Check sheet for the modelled part. Datum: model origin and axes. Units: mm. A direction names the side the tool comes from. Give positions to 0.01 mm unless a question says otherwise; leave off trailing zeros. Write each loop counter-clockwise with the first axis right and the second up, starting at its lowest first coordinate (ties: lowest second). Pieces come first, ordered by that corner, then holes. Notation, with made-up numbers: (-10, -36.75) -> (0, -36.75) arc R16 ccw to (0, -17.75) -> close; hole circle Ø7 at (84.25, 6). An arc over 180 degrees is marked (long way). Use a Markdown table: item, result. Add a question column.
1. Cross-section at A-A (x = 2). Enter the section's corners in (y, z).
2. Release check for a two-part mould opening along Y. For faces 4 (the cylindrical face through (4.5, 23.6, 3.6)), 5 (the flat face through (0.1, 0, 4.3)), 6 (the cylindrical face through (4.5, 23.6, -3.7)), 7 (the cylindrical face through (-0.1, 26.1, 2.5)) record: released by +Y, released by -Y, zero draft, split by the parting line, or undercut.
3. Set-up check for faces 1 (the flat face through (0, 17.5, 3)), 2 (the cylindrical face through (0.1, 26.1, -2.5)), 3 (the flat face through (6, 18, -0.25)): record each of +Z, -Z, +X, -X, +Y, -Y from which the full face is reachable in a straight line by a thin tool's end or side.
4. Cross-section at D-D (y = 14). Enter the section's corners in (x, z), then the cut area to 3 significant figures.
5. Cross-section at C-C (z = 8). Enter the section's corners in (x, y).
6. Cross-section at B-B (y = 31.5). Enter the section's corners in (x, z).
7. Scan lines: probe 1 along X at (y, z) = (3.5, 3.25); probe 2 along Y at (x, z) = (7.5, -2.75); probe 3 along Z at (x, y) = (4.5, 10.5). Record each from-to range of solid material in increasing order. Write a range as [from, to].
8. Gauge pin test, flat ends, axial feed: P1, Ø3.5, axis at x = 6.5, y = 3.5, coming from the +Z side; P2, Ø10, axis at x = 7.5, y = 29, coming from the +Z side; P3, Ø1.9, axis at x = 1.5, z = 3, coming from the -Y side; P4, Ø1.3, axis at x = -3.5, y = 15.5, coming from the +Z side. Record the tip position at first contact, or that the pin passes through.
from build123d import *

# Parameters (mm, degrees)
SKETCH1_R               = 10
BOSS_EXTRUDE1_DEPTH     = 35
CUT_EXTRUDE1_DEPTH      = 38.749172176
CUT_EXTRUDE1_DEPTH_BACK = 38.749172176
SKETCH2_R               = 2.5
SKETCH3_R               = 4
CUT_EXTRUDE2_DEPTH      = 17.5
CUT_EXTRUDE3_DEPTH      = 38.749172176
CUT_EXTRUDE3_DEPTH_BACK = 38.749172176
SKETCH4_W               = 15
SKETCH4_H               = 0.5
CUT_EXTRUDE4_DEPTH      = 38.749172176
CUT_EXTRUDE4_DEPTH_BACK = 38.749172176
SKETCH5_R               = 2


with BuildPart() as part:
    # Sketch1 → Boss-Extrude1 (new body)
    with BuildSketch(Plane(origin=(0, 0, 0), x_dir=(1, 0, 0), z_dir=(0, 1, 0))):
        with Locations(Location((0, 0, 0), (0, 0, 270))):
            Circle(SKETCH1_R)
    extrude(amount=BOSS_EXTRUDE1_DEPTH)

    # Sketch2 → Cut-Extrude1 (cut, two sides: drawn at the far end of the back side and taken through both)
    with BuildSketch(Plane(origin=(0, 35, 0), x_dir=(1, 0, 0), z_dir=(0, 1, 0)).offset(-CUT_EXTRUDE1_DEPTH_BACK)):
        with Locations(Location((0, 0, 0), (0, 0, 270))):
            Circle(SKETCH2_R)
    extrude(amount=CUT_EXTRUDE1_DEPTH + CUT_EXTRUDE1_DEPTH_BACK, mode=Mode.SUBTRACT)

    # Sketch3 → Cut-Extrude2 (cut)
    with BuildSketch(Plane.XZ):
        with Locations(Location((0, 0, 0), (0, 0, 270))):
            Circle(SKETCH3_R)
    extrude(amount=-CUT_EXTRUDE2_DEPTH, mode=Mode.SUBTRACT)

    # Sketch4 → Cut-Extrude3 (cut, two sides: drawn at the far end of the back side and taken through both)
    with BuildSketch(Plane.XZ.offset(-CUT_EXTRUDE3_DEPTH_BACK)):
        with Locations((2.5, 0)):
            Rectangle(SKETCH4_W, SKETCH4_H)
    extrude(amount=CUT_EXTRUDE3_DEPTH + CUT_EXTRUDE3_DEPTH_BACK, mode=Mode.SUBTRACT)

    # Sketch5 → Cut-Extrude4 (cut, two sides: drawn at the far end of the back side and taken through both)
    with BuildSketch(Plane.XY.offset(-CUT_EXTRUDE4_DEPTH_BACK)):
        with Locations((6.496874512, 31.5)):
            Circle(SKETCH5_R)
        with Locations((6.496874512, 23.5)):
            Circle(SKETCH5_R)
        with Locations((6.496874512, 11.5)):
            Circle(SKETCH5_R)
        with Locations((6.496874512, 3.5)):
            Circle(SKETCH5_R)
    extrude(amount=CUT_EXTRUDE4_DEPTH + CUT_EXTRUDE4_DEPTH_BACK, mode=Mode.SUBTRACT)


solid = part.part
Worked answers:
| question | item | result |
|---|---|---|
| 1 | outline | (0, -9.8) -> (35, -9.8) -> (35, -1.5) -> (17.5, -1.5) -> (17.5, -3.46) -> (0, -3.46) -> close; (0, 3.46) -> (17.5, 3.46) -> (17.5, 1.5) -> (35, 1.5) -> (35, 9.8) -> (0, 9.8) -> close |
| 2 | face 4 | undercut |
| 2 | face 5 | released by -Y |
| 2 | face 6 | undercut |
| 2 | face 7 | zero draft |
| 3 | face 1 | -Y |
| 3 | face 2 | +Y, -Y |
| 3 | face 3 | +X, +Y, -Y |
| 4 | outline | (-5, -0.25) -> (-5, 0.25) -> (-3.99, 0.25) arc R4 cw to (3.99, 0.25) -> (10, 0.25) arc R10 ccw (long way) to (10, -0.25) -> (3.99, -0.25) arc R4 cw to (-3.99, -0.25) -> close |
| 4 | area | 260 mm² |
| 5 | outline | (-6, 0) -> (6, 0) -> (6, 1.56) arc R2 cw to (6, 5.44) -> (6, 9.56) arc R2 cw to (6, 13.44) -> (6, 21.56) arc R2 cw to (6, 25.44) -> (6, 29.56) arc R2 cw to (6, 33.44) -> (6, 35) -> (-6, 35) -> close |
| 6 | outline | (-5, -0.25) -> (-5, 0.25) -> (-2.49, 0.25) arc R2.5 cw to (2.49, 0.25) -> (4.5, 0.25) -> (4.5, 8.93) arc R10 ccw (long way) to (4.5, -8.93) -> (4.5, -0.25) -> (2.49, -0.25) arc R2.5 cw to (-2.49, -0.25) -> close; (8.5, -5.27) arc R10 ccw to (10, -0.25) -> (8.5, -0.25) -> close; (8.5, 0.25) -> (10, 0.25) arc R10 ccw to (8.5, 5.27) -> close |
| 7 | probe 1 | x = [-9.46, -2.33], [2.33, 4.5], [8.5, 9.46] |
| 7 | probe 2 | y = [0, 1.77], [5.23, 9.77], [13.23, 21.77], [25.23, 29.77], [33.23, 35] |
| 7 | probe 3 | z = [-8.93, -0.25], [0.25, 8.93] |
| 8 | P1 | passes through |
| 8 | P2 | stops at z = 9.68 |
| 8 | P3 | stops at y = 0 |
| 8 | P4 | stops at z = 9.59 |
